Geometry check sheet. Reference: the model listing, model coordinates, mm. Face numbers are marked on the shaded views. A direction names the side the tool comes from. Round coordinates to 2 decimals unless told otherwise and drop trailing zeros. Order: outer loops, then holes, each group sorted by start corner. A loop starts at its lowest first (then second) coordinate and runs counter-clockwise, first axis right, second up. Notation, with made-up numbers: (24, 52.25) - (80, 52.25) arc R16 ccw to (80, 68.25) - close; hole circle Ø6 at (80, -0.5). An arc over 180 degrees is marked (long way). Answer as CSV lines item,"result". Start each with the question number.
```python
from build123d import *

# Parameters (mm, degrees)
SKETCH1_R           = 10
BOSS_EXTRUDE1_DEPTH = 245.53
SKETCH2_R           = 10.5
BOSS_EXTRUDE2_DEPTH = 11
SKETCH3_R           = 15
BOSS_EXTRUDE3_DEPTH = 22
SKETCH4_W           = 32
SKETCH4_H           = 32
BOSS_EXTRUDE4_DEPTH = 61
SKETCH5_W           = 50
SKETCH5_H           = 16
CUT_EXTRUDE1_DEPTH  = 58
SKETCH6_R           = 8
CUT_EXTRUDE2_DEPTH  = 58
FILLET1_R           = 10


with BuildPart() as part:
    # Sketch1 → Boss-Extrude1 (new body)
    with BuildSketch(Plane.XY):
        with Locations(Location((0, 0, 0), (0, 0, 180))):
            Circle(SKETCH1_R)
    extrude(amount=BOSS_EXTRUDE1_DEPTH)

    # Sketch2 → Boss-Extrude2 (add)
    with BuildSketch(Plane.XY.offset(245.53)):
        Circle(SKETCH2_R)
    extrude(amount=BOSS_EXTRUDE2_DEPTH)

    # Sketch3 → Boss-Extrude3 (add)
    with BuildSketch(Plane.XY.offset(256.53)):
        Circle(SKETCH3_R)
    extrude(amount=BOSS_EXTRUDE3_DEPTH)

    # Sketch4 → Boss-Extrude4 (add)
    with BuildSketch(Plane.XY.offset(278.53)):
        Rectangle(SKETCH4_W, SKETCH4_H)
    extrude(amount=BOSS_EXTRUDE4_DEPTH)

    # Sketch5 → Cut-Extrude1 (cut)
    with BuildSketch(Plane.ZY.offset(16)):
        with Locations((314.53, 0)):
            Rectangle(SKETCH5_W, SKETCH5_H)
    extrude(amount=-CUT_EXTRUDE1_DEPTH, mode=Mode.SUBTRACT)

    # Sketch6 → Cut-Extrude2 (cut)
    with BuildSketch(Plane(origin=(0, 16, 0), x_dir=(1, 0, 0), z_dir=(0, 1, 0))):
        with Locations(Location((0, -321.53, 0), (0, 0, 270))):
            Circle(SKETCH6_R)
    extrude(amount=-CUT_EXTRUDE2_DEPTH, mode=Mode.SUBTRACT)

    # Fillet1
    fillet1_edges = [part.edges().sort_by_distance(p)[0] for p in [
        (16, -12, 339.53),
        (-16, 12, 339.53),
        (16, 12, 339.53),
        (-16, -12, 339.53),
    ]]
    fillet(fillet1_edges, radius=FILLET1_R)


solid = part.part
```
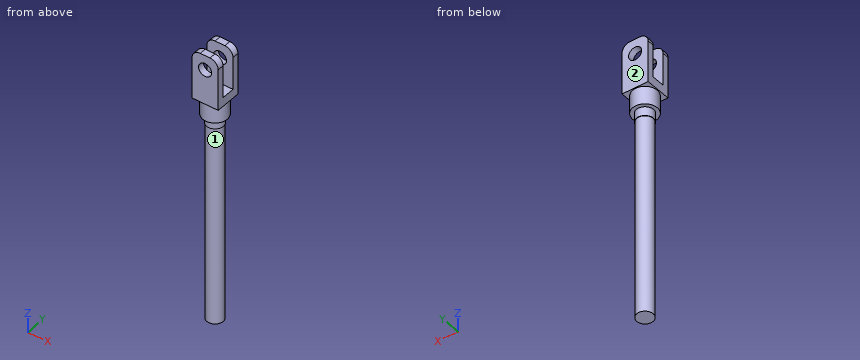
1. Go/stop test with flat-tipped pins: pin 1 Ø4 at (x, z) = (-12.5, 199) entering from -Y; pin 2 Ø5 at (x, y) = (-3, -2.5) entering from +Z; pin 3 Ø6 at (x, z) = (11, 117) entering from +Y; pin 4 Ø12 at (x, z) = (-10.5, 132.5) entering from +Y. Record where each tip stops, or that it passes through.
2. Section check D-D on z = 110. Record the boundary of the cut face in (x, y), plus the area to 3 significant figures.
3. Section check C-C on y = 0. Record the boundary of the cut face in (x, z), plus the area to 3 significant figures.
4. Access from +Z, -Z, +X, -X, +Y, -Y to the whole of each face (thin tool, end or side, straight path). Record for the marked faces 1 and 2.
5. Section check A-A on x = 0. Record the boundary of the cut face in (y, z), plus the area to 3 significant figures.
6. Section check B-B on z = 321.53. Record the boundary of the cut face in (x, y), plus the area to 3 significant figures.
7. Thickness scan on probe 1 along X at (y, z) = (12, 321.53); probe 2 along Z at (x, y) = (-6, 0.5); probe 3 along X at (y, z) = (0.5, 128.5). Record the ranges inside material, lowest first.
Numbers:
1,pin 1,"passes through"
1,pin 2,"stops at z = 289.53"
1,pin 3,"stops at y = 6"
1,pin 4,"stops at y = 8.93"
2,outline,"circle Ø20 at (0, 0)"
2,area,"314 mm2"
3,outline,"(-16, 278.53) - (-15, 278.53) - (-15, 256.53) - (-10.5, 256.53) - (-10.5, 245.53) - (-10, 245.53) - (-10, 0) - (10, 0) - (10, 245.53) - (10.5, 245.53) - (10.5, 256.53) - (15, 256.53) - (15, 278.53) - (16, 278.53) - (16, 289.53) - (-16, 289.53) - close"
3,area,"6,150 mm2"
4,face 1,"-Z"
4,face 2,"+Z, -Z, +X, -X, +Y"
5,outline,"(-16, 278.53) - (-15, 278.53) - (-15, 256.53) - (-10.5, 256.53) - (-10.5, 245.53) - (-10, 245.53) - (-10, 0) - (10, 0) - (10, 245.53) - (10.5, 245.53) - (10.5, 256.53) - (15, 256.53) - (15, 278.53) - (16, 278.53) - (16, 313.53) - (8, 313.53) - (8, 289.53) - (-8, 289.53) - (-8, 313.53) - (-16, 313.53) - close; (-16, 329.53) - (-8, 329.53) - (-8, 339.53) - (-16, 339.53) - close; (8, 329.53) - (16, 329.53) - (16, 339.53) - (8, 339.53) - close"
5,area,"6,700 mm2"
6,outline,"(-16, -16) - (-8, -16) - (-8, -8) - (-16, -8) - close; (-16, 8) - (-8, 8) - (-8, 16) - (-16, 16) - close; (8, -16) - (16, -16) - (16, -8) - (8, -8) - close; (8, 8) - (16, 8) - (16, 16) - (8, 16) - close"
6,area,"256 mm2"
7,probe 1,"x = -16 to -8, 8 to 16"
7,probe 2,"z = 0 to 289.53"
7,probe 3,"x = -9.99 to 9.99"
